```python
from build123d import *

# Parameters (mm, degrees)
BOSS_EXTRUDE1_DEPTH = 40


with BuildPart() as part:
    # Sketch1 → Boss-Extrude1 (new body)
    with BuildSketch(Plane.XY):
        with BuildLine():
            Line((-18.982831897, 2.385797253), (-16.128175583, 5.240453568))
            ThreePointArc((-16.128175583, 5.240453568), (-14.388813512, 1.507034758), (-14.671071516, -2.601995157))
            ThreePointArc((-14.671071516, -2.601995157), (-16.108631881, -3.917504194), (-17.983207135, -3.385422015))
            Line((-17.983207135, -3.385422015), (-18.982831897, -2.385797253))
            ThreePointArc((-18.982831897, -2.385797253), (-19.49479618, -3.00520382), (-20.114202747, -3.517168103))
            Line((-20.114202747, -3.517168103), (-16.01728135, -7.6140895))
            Line((-16.01728135, -7.6140895), (16.01728135, -7.6140895))
            Line((16.01728135, -7.6140895), (20.114202747, -3.517168103))
            ThreePointArc((20.114202747, -3.517168103), (19.49479618, -3.00520382), (18.982831897, -2.385797253))
            Line((18.982831897, -2.385797253), (17.983207135, -3.385422015))
            ThreePointArc((17.983207135, -3.385422015), (16.108631881, -3.917504194), (14.671071516, -2.601995157))
            ThreePointArc((14.671071516, -2.601995157), (14.388813512, 1.507034758), (16.128175583, 5.240453568))
            Line((16.128175583, 5.240453568), (18.982831897, 2.385797253))
            ThreePointArc((18.982831897, 2.385797253), (19.49479618, 3.00520382), (20.114202747, 3.517168103))
            Line((20.114202747, 3.517168103), (17.259546432, 6.371824417))
            ThreePointArc((17.259546432, 6.371824417), (22.5, 8.25), (27.740453568, 6.371824417))
            Line((27.740453568, 6.371824417), (24.885797253, 3.517168103))
            ThreePointArc((24.885797253, 3.517168103), (25.50520382, 3.00520382), (26.017168103, 2.385797253))
            Line((26.017168103, 2.385797253), (28.871824417, 5.240453568))
            ThreePointArc((28.871824417, 5.240453568), (30.611186488, 1.507034758), (30.328928484, -2.601995157))
            ThreePointArc((30.328928484, -2.601995157), (28.891368119, -3.917504194), (27.016792865, -3.385422015))
            Line((27.016792865, -3.385422015), (26.017168103, -2.385797253))
            ThreePointArc((26.017168103, -2.385797253), (25.50520382, -3.00520382), (24.885797253, -3.517168103))
            Line((24.885797253, -3.517168103), (28.98271865, -7.6140895))
            ThreePointArc((28.98271865, -7.6140895), (31.884585633, 3.453918427), (22.5, 10))
            Line((22.5, 10), (-22.5, 10))
            ThreePointArc((-22.5, 10), (-31.884585633, 3.453918427), (-28.98271865, -7.6140895))
            Line((-28.98271865, -7.6140895), (-24.885797253, -3.517168103))
            ThreePointArc((-24.885797253, -3.517168103), (-25.50520382, -3.00520382), (-26.017168103, -2.385797253))
            Line((-26.017168103, -2.385797253), (-27.016792865, -3.385422015))
            ThreePointArc((-27.016792865, -3.385422015), (-28.891368119, -3.917504194), (-30.328928484, -2.601995157))
            ThreePointArc((-30.328928484, -2.601995157), (-30.611186488, 1.507034758), (-28.871824417, 5.240453568))
            Line((-28.871824417, 5.240453568), (-26.017168103, 2.385797253))
            ThreePointArc((-26.017168103, 2.385797253), (-25.50520382, 3.00520382), (-24.885797253, 3.517168103))
            Line((-24.885797253, 3.517168103), (-27.740453568, 6.371824417))
            ThreePointArc((-27.740453568, 6.371824417), (-22.5, 8.25), (-17.259546432, 6.371824417))
            Line((-17.259546432, 6.371824417), (-20.114202747, 3.517168103))
            ThreePointArc((-20.114202747, 3.517168103), (-19.49479618, 3.00520382), (-18.982831897, 2.385797253))
        make_face()
    extrude(amount=BOSS_EXTRUDE1_DEPTH)

    # Sketch3 → Cut-Revolve1 (revolve, cut)
    with BuildSketch(Plane.XY.offset(40)):
        Polygon((12, 8), (10, 8), (10, 6), (14, 6), (14, 8), align=None)
        Polygon((-14, 8), (-12, 8), (-10, 8), (-10, 6), (-14, 6), align=None)
    cut_revolve1 = revolve(axis=Axis((-22.5, 10, 40), (-1, 0, 0)), mode=Mode.SUBTRACT)

    # Mirror1: Cut-Revolve1 across plane
    add(cut_revolve1.mirror(Plane.XY.offset(20)), mode=Mode.SUBTRACT)


solid = part.part
```
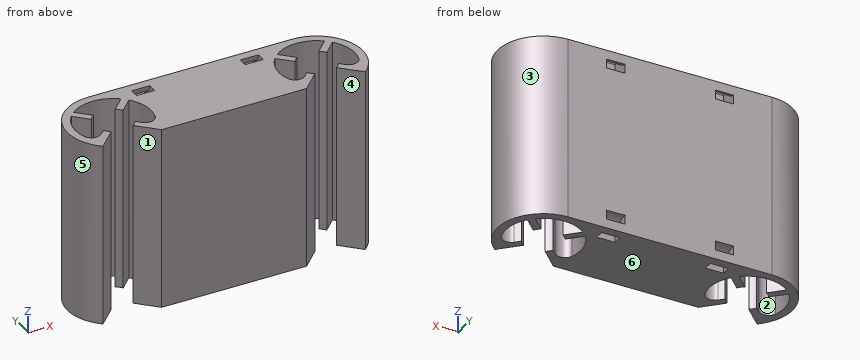
Geometry check sheet. Reference: the model listing, model coordinates, mm. Face numbers are marked on the shaded views. A direction names the side the tool comes from. Coordinates: 2 decimals unless noted, no trailing zeros. Loops run counter-clockwise (first coordinate to the right, second up) from the corner with the lowest first, then second, coordinate; pieces in that order, holes last.
Item 1: Release check for a two-part mould opening along X. For the marked faces 4, 5 and 6 record: released by +X, released by -X, zero draft, split by the parting line, or undercut.
Item 2: Go/stop test with flat-tipped pins: pin 1 Ø4.5 at (y, z) = (9, 1) entering from +X; pin 2 Ø1.2 at (y, z) = (7, 37.5) entering from +X; pin 3 Ø5 at (y, z) = (4, 27) entering from +X. Record where each tip stops, or that it passes through.
Item 3: Thickness scan on line 1 (X direction, y = 6.75, z = 18); line 2 (X direction, y = -7, z = 34); line 3 (Y direction, x = 18, z = 23). Record the ranges inside material, lowest first.
Item 4: Access from +Z, -Z, +X, -X, +Y, -Y to the whole of each face (thin tool, end or side, straight path). Record for the marked faces 1, 2 and 3.
Item 5: Sectioned sample at A-A, the plane y = -0.25. Record the boundary of the cut face in (x, z), then the cut area to 3 significant figures.
Item 6: Sectioned sample at B-B, the plane y = -5.75. Record the boundary of the cut face in (x, z).
Check result:
1. face 4: undercut
1. face 5: released by -X
1. face 6: zero draft
2. pin 1: stops at x = 29.88
2. pin 2: stops at x = 30.18
2. pin 3: stops at x = 32.39
3. line 1: x = -29.88 to -27.24, -17.76 to 17.76, 27.24 to 29.88
3. line 2: x = -29.64 to -28.37, -16.63 to 16.63, 28.37 to 29.64
3. line 3: y = -5.63 to -3.37, 3.37 to 5.63, 6.91 to 10
4. face 1: +Z, -Z, -Y
4. face 2: +Z, -Z
4. face 3: +Z, -Z, +X
5. outline: (-32.5, 0) - (-30.75, 0) - (-30.75, 40) - (-32.5, 40) - close; (-14.25, 0) - (14.25, 0) - (14.25, 40) - (-14.25, 40) - close; (30.75, 0) - (32.5, 0) - (32.5, 40) - (30.75, 40) - close
5. area: 1,280 mm2
6. outline: (-30.68, 0) - (-27.12, 0) - (-27.12, 40) - (-30.68, 40) - close; (-17.88, 0) - (17.88, 0) - (17.88, 40) - (-17.88, 40) - close; (27.12, 0) - (30.68, 0) - (30.68, 40) - (27.12, 40) - close
